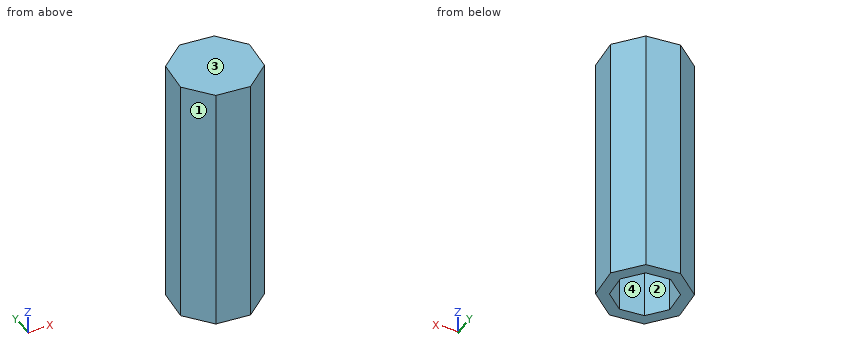
from build123d import *

# Parameters (mm, degrees)
RESSALTO_EXTRUS_O1_DEPTH = 100
CORTE_EXTRUS_O1_DEPTH    = 20


with BuildPart() as part:
    # Esboço2 → Ressalto-extrusão1 (new body)
    with BuildSketch(Plane.XY):
        Polygon((15.207285045, -8.286201641), (16.612403749, 4.893945008), (8.286201641, 15.207285045), (-4.893945008, 16.612403749), (-15.207285045, 8.286201641), (-16.612403749, -4.893945008), (-8.286201641, -15.207285045), (4.893945008, -16.612403749), align=None)
    extrude(amount=RESSALTO_EXTRUS_O1_DEPTH)

    # Esboço1 → Corte-extrusão1 (cut)
    with BuildSketch(Plane.XY):
        Polygon((10.930236126, -5.95570743), (11.940165195, 3.517522974), (5.95570743, 10.930236126), (-3.517522974, 11.940165195), (-10.930236126, 5.95570743), (-11.940165195, -3.517522974), (-5.95570743, -10.930236126), (3.517522974, -11.940165195), align=None)
    extrude(amount=CORTE_EXTRUS_O1_DEPTH, mode=Mode.SUBTRACT)


solid = part.part
Here's how the part is built. I have some questions about the finished solid (model axes, mm). Face numbers are marked on the shaded views. Coordinates: 2 decimals unless noted, no trailing zeros. Loops run counter-clockwise (first coordinate to the right, second up) from the corner with the lowest first, then second, coordinate; pieces in that order, holes last.
1. Imagine slicing it at B-B, the plane z = 41. Please give me the cut outline in (x, y), and give its area (3 significant figures).
2. Imagine slicing it at D-D, the plane y = -14. Please give me the cut outline in (x, z).
3. If we mould it in two halves opening along Y, with no side actions, what happens to the marked faces 1, 2, 3 and 4? For each: pulls with the +Y half, pulls with the -Y half, needs draft (parallel to the pull), parting line crosses it, or undercut.
4. Imagine slicing it at A-A, the plane z = 10.5. Please give me the cut outline in (x, y), and give its area (3 significant figures).
5. Imagine slicing it at C-C, the plane x = -7. Please give me the cut outline in (y, z).
6. I need wall thicknesses on L1, parallel to Z at x = -3.5, y = 2; L2, parallel to Y at x = 4, z = 15.5; L3, parallel to X at y = 2, z = 67. Which ranges of each line are inside material? Lowest first, please.
7. For P1, Ø6, axis at x = -2.5, z = 73.5, coming from the -Y side; P2, Ø8, axis at y = -1, z = 42, coming from the +X side; P3, Ø1, axis at y = 10, z = 34, coming from the +X side, each with a flat end and sliding along its axis, tell me the tip position at first contact or that it passes through.
Taken from the geometry:
1. outline: (-16.61, -4.89) - (-8.29, -15.21) - (4.89, -16.61) - (15.21, -8.29) - (16.61, 4.89) - (8.29, 15.21) - (-4.89, 16.61) - (-15.21, 8.29) - close
1. area: 848 mm2
2. outline: (-9.26, 0) - (8.13, 0) - (8.13, 100) - (-9.26, 100) - close
3. face 1: pulls with the -Y half
3. face 2: undercut
3. face 3: needs draft
3. face 4: undercut
4. outline: (-16.61, -4.89) - (-8.29, -15.21) - (4.89, -16.61) - (15.21, -8.29) - (16.61, 4.89) - (8.29, 15.21) - (-4.89, 16.61) - (-15.21, 8.29) - close; hole (-11.94, -3.52) - (-5.96, -10.93) - (3.52, -11.94) - (10.93, -5.96) - (11.94, 3.52) - (5.96, 10.93) - (-3.52, 11.94) - (-10.93, 5.96) - close
4. area: 410 mm2
5. outline: (-15.34, 0) - (-9.64, 0) - (-9.64, 20) - (9.13, 20) - (9.13, 0) - (14.91, 0) - (14.91, 100) - (-15.34, 100) - close
6. L1: z = 20 to 100
6. L2: y = -16.52 to -11.55, 11.14 to 15.66
6. L3: x = -15.88 to 16.3
7. P1: stops at y = -16.14
7. P2: stops at x = 16.41
7. P3: stops at x = 12.89
